from build123d import *

# Parameters (mm, degrees)
ESQUISSE1_W             = 40
ESQUISSE1_H             = 18
BOSS_EXTRU_1_DEPTH      = 3
ESQUISSE2_W             = 3
ESQUISSE2_H             = 18
BOSS_EXTRU_2_DEPTH      = 37
ESQUISSE3_R             = 1.5
ENL_V_MAT_EXTRU_1_DEPTH = 58.384666942
ESQUISSE4_R             = 2
ENL_V_MAT_EXTRU_2_DEPTH = 58.384666942
ENL_V_MAT_EXTRU_3_DEPTH = 1.5


with BuildPart() as part:
    # Esquisse1 → Boss.-Extru.1 (new body)
    with BuildSketch(Plane.XY):
        with Locations((20, 9)):
            Rectangle(ESQUISSE1_W, ESQUISSE1_H)
    extrude(amount=BOSS_EXTRU_1_DEPTH)

    # Esquisse2 → Boss.-Extru.2 (add)
    with BuildSketch(Plane.XY.offset(3)):
        with Locations((1.5, 9)):
            Rectangle(ESQUISSE2_W, ESQUISSE2_H)
    extrude(amount=BOSS_EXTRU_2_DEPTH)

    # Esquisse3 → Enlèv. mat.-Extru.1 (cut, through all)
    with BuildSketch(Plane.XY.offset(3)):
        with Locations((14.5, 15)):
            Circle(ESQUISSE3_R)
        with Locations((29.5, 15)):
            Circle(ESQUISSE3_R)
        with Locations((14.5, 5)):
            Circle(ESQUISSE3_R)
        with Locations((29.5, 5)):
            Circle(ESQUISSE3_R)
    extrude(amount=-ENL_V_MAT_EXTRU_1_DEPTH, mode=Mode.SUBTRACT)

    # Esquisse4 → Enlèv. mat.-Extru.2 (cut, through all)
    with BuildSketch(Plane(origin=(3, 0, 0), x_dir=(0, 0, -1), z_dir=(1, 0, 0))):
        with Locations(Location((-28, 8, 0), (0, 0, 90))):
            Circle(ESQUISSE4_R)
        with Locations(Location((-13, 8, 0), (0, 0, 90))):
            Circle(ESQUISSE4_R)
    extrude(amount=-ENL_V_MAT_EXTRU_2_DEPTH, mode=Mode.SUBTRACT)

    # Esquisse5 → Enlèv. mat.-Extru.3 (cut)
    with BuildSketch(Plane.XY.offset(3)):
        Polygon((12.854551733, 7.85), (11.209103466, 5), (12.854551733, 2.15), (16.145448267, 2.15), (17.790896534, 5), (16.145448267, 7.85), align=None)
        Polygon((27.854551733, 17.85), (26.209103466, 15), (27.854551733, 12.15), (31.145448267, 12.15), (32.790896534, 15), (31.145448267, 17.85), align=None)
        Polygon((27.854551733, 7.85), (26.209103466, 5), (27.854551733, 2.15), (31.145448267, 2.15), (32.790896534, 5), (31.145448267, 7.85), align=None)
        Polygon((12.854551733, 17.85), (11.209103466, 15), (12.854551733, 12.15), (16.145448267, 12.15), (17.790896534, 15), (16.145448267, 17.85), align=None)
    extrude(amount=-ENL_V_MAT_EXTRU_3_DEPTH, mode=Mode.SUBTRACT)


solid = part.part
The listing builds one solid part. Answer for the finished solid, in the listing's coordinates (mm). A direction names the side the tool comes from. Give positions to 0.01 mm unless a question says otherwise; leave off trailing zeros. Loops run counter-clockwise (first coordinate to the right, second up) from the corner with the lowest first, then second, coordinate; pieces in that order, holes last. Notation, with made-up numbers: (14, 84) - (21, 84) arc R30 ccw to (21, 117) - close; hole circle Ø4 at (87, 41). An arc over 180 degrees is marked (long way). Answer as a JSON object with one key per item and string values.
1. A cutting plane is placed at A-A (x = 29.5). Write down the section's boundary in (y, z).
Determined:
{"outline": "(0, 0) - (3.5, 0) - (3.5, 1.5) - (2.15, 1.5) - (2.15, 3) - (0, 3) - close; (6.5, 0) - (13.5, 0) - (13.5, 1.5) - (12.15, 1.5) - (12.15, 3) - (7.85, 3) - (7.85, 1.5) - (6.5, 1.5) - close; (16.5, 0) - (18, 0) - (18, 3) - (17.85, 3) - (17.85, 1.5) - (16.5, 1.5) - close"}
2. A cutting plane is placed at D-D (z = 5). Write down the section's boundary in (x, y), then the cut area to 3 significant figures.
Determined:
{"outline": "(0, 0) - (3, 0) - (3, 18) - (0, 18) - close", "area": "54.0 mm²"}
3. A cutting plane is placed at C-C (x = 17). Write down the section's boundary in (y, z), then the cut area to 3 significant figures.
Determined:
{"outline": "(0, 0) - (18, 0) - (18, 3) - (16.37, 3) - (16.37, 1.5) - (13.63, 1.5) - (13.63, 3) - (6.37, 3) - (6.37, 1.5) - (3.63, 1.5) - (3.63, 3) - (0, 3) - close", "area": "45.8 mm²"}
4. Flat-ended cylindrical pins translate along their axes: pin 1 Ø3 at (x, y) = (16, 14.5) entering from +Z; pin 2 Ø8 at (x, y) = (12, 11.5) entering from -Z; pin 3 Ø4 at (y, z) = (2, 24.5) entering from +X; pin 4 Ø2.5 at (x, y) = (14.5, 5) entering from +Z. Find the tip coordinate at first contact, or state that the pin passes through.
Determined:
{"pin 1": "z = 3", "pin 2": "z = 0", "pin 3": "x = 3", "pin 4": "through"}
5. For a pull along Z with two mould halves and no side action, classify faces 1 (the cylindrical face through (1.521, 6.526, 14.352)), 2 (the flat face through (16, 6, 1.5)), 3 (the flat face through (27.02, 13.595, 2.26)) as pulls with the +Z half, pulls with the -Z half, needs draft (parallel to the pull), parting line crosses it, or undercut.
Determined:
{"face 1": "undercut", "face 2": "pulls with the +Z half", "face 3": "needs draft"}
6. For faces 4 (the flat face through (0, 9, 20)), 5 (the flat face through (27.02, 3.595, 2.26)), determine the directions among +Z, -Z, +X, -X, +Y, -Y from which every point of the face is accessible in a straight line to the end or side of a thin tool.
Determined:
{"face 4": "+Z, -Z, -X, +Y, -Y", "face 5": "+Z"}
7. A cutting plane is placed at B-B (z = 28). Write down the section's boundary in (x, y).
Determined:
{"outline": "(0, 0) - (3, 0) - (3, 6) - (0, 6) - close; (0, 10) - (3, 10) - (3, 18) - (0, 18) - close"}
8. Find the intervals of material crossed by L1, parallel to Y at x = 29.5, z = 0.3; L2, parallel to Z at x = 1.7, y = 8; L3, parallel to Z at x = 29, y = 10.5, in increasing order. Write a range as [from, to].
Determined:
{"L1": "[0, 3.5], [6.5, 13.5], [16.5, 18]", "L2": "[0, 11], [15, 26], [30, 40]", "L3": "[0, 3]"}
